Here's how the part is built. I have some questions about the finished solid (model axes, mm). Face numbers are marked on the shaded views. A direction names the side the tool comes from. Give positions to 0.01 mm unless a question says otherwise; leave off trailing zeros. Order: outer loops, then holes, each group sorted by start corner. A loop starts at its lowest first (then second) coordinate and runs counter-clockwise, first axis right, second up. Notation, with made-up numbers: (70, 52) - (96, 52) arc R27 cw to (96, 90) - close; hole circle Ø11 at (72.25, 69). An arc over 180 degrees is marked (long way). One line per question, with ' | ' between items.
from build123d import *

# Parameters (mm, degrees)
SKETCH1_R               = 6.477
BOSS_EXTRUDE2_DEPTH     = 12.7
CUT_EXTRUDE1_DEPTH      = 2.032
CUT_EXTRUDE1_TAPER      = 15
CUT_EXTRUDE2_DEPTH      = 2.032
CUT_EXTRUDE2_TAPER      = 15
SKETCH6_R               = 15.308441
SKETCH6_R_2             = 10.16
CUT_EXTRUDE3_DEPTH      = 112.76
CUT_EXTRUDE3_DEPTH_BACK = 11.16


with BuildPart() as part:
    # Sketch1 → Boss-Extrude2 (new body)
    with BuildSketch(Plane.XY):
        with BuildLine():
            Line((-10.16, 0), (-10.16, 12.7))
            Line((-10.16, 12.7), (-3.181447, 28.448))
            Line((-3.181447, 28.448), (-3.181447, 91.950959))
            ThreePointArc((-3.181447, 91.950959), (0, 111.76), (3.181447, 91.950959))
            Line((3.181447, 91.950959), (3.181447, 28.448))
            Line((3.181447, 28.448), (10.16, 12.7))
            Line((10.16, 12.7), (10.16, 0))
            ThreePointArc((10.16, 0), (0, -10.16), (-10.16, 0))
        make_face()
        Circle(SKETCH1_R, mode=Mode.SUBTRACT)
        with Locations((0, 101.6)):
            Circle(SKETCH1_R, mode=Mode.SUBTRACT)
    extrude(amount=BOSS_EXTRUDE2_DEPTH)

    # Sketch3 → Cut-Extrude1 (cut)
    with BuildSketch(Plane.XY.offset(12.7)):
        with BuildLine():
            ThreePointArc((-0.895447, 89.408), (-1.973078, 88.961631), (-2.419447, 87.884))
            Line((-2.419447, 87.884), (-2.419447, 32.766))
            ThreePointArc((-2.419447, 32.766), (-1.973078, 31.688369), (-0.895447, 31.242))
            Line((-0.895447, 31.242), (0.895447, 31.242))
            ThreePointArc((0.895447, 31.242), (1.973078, 31.688369), (2.419447, 32.766))
            Line((2.419447, 32.766), (2.419447, 87.884))
            ThreePointArc((2.419447, 87.884), (1.973078, 88.961631), (0.895447, 89.408))
            Line((0.895447, 89.408), (-0.895447, 89.408))
        make_face()
    extrude(amount=-CUT_EXTRUDE1_DEPTH, taper=CUT_EXTRUDE1_TAPER, mode=Mode.SUBTRACT)

    # Sketch5 → Cut-Extrude2 (cut)
    with BuildSketch(Plane(origin=(0, 0, 0), x_dir=(-1, 0, 0), z_dir=(0, 0, -1))):
        with BuildLine():
            ThreePointArc((-0.895447, 89.408), (-1.973078, 88.961631), (-2.419447, 87.884))
            Line((-2.419447, 87.884), (-2.419447, 32.766))
            ThreePointArc((-2.419447, 32.766), (-1.973078, 31.688369), (-0.895447, 31.242))
            Line((-0.895447, 31.242), (0.895447, 31.242))
            ThreePointArc((0.895447, 31.242), (1.973078, 31.688369), (2.419447, 32.766))
            Line((2.419447, 32.766), (2.419447, 87.884))
            ThreePointArc((2.419447, 87.884), (1.973078, 88.961631), (0.895447, 89.408))
            Line((0.895447, 89.408), (-0.895447, 89.408))
        make_face()
    extrude(amount=-CUT_EXTRUDE2_DEPTH, taper=CUT_EXTRUDE2_TAPER, mode=Mode.SUBTRACT)

    # Sketch6 → Cut-Extrude3 (cut, two sides)
    with BuildSketch(Plane(origin=(0, 0, 0), x_dir=(1, 0, 0), z_dir=(0, 1, 0))) as cut_extrude3_sk:
        with Locations((0, -6.388373)):
            Circle(SKETCH6_R)
        with Locations((0, -6.388373)):
            Circle(SKETCH6_R_2, mode=Mode.SUBTRACT)
    extrude(amount=CUT_EXTRUDE3_DEPTH, mode=Mode.SUBTRACT)
    extrude(cut_extrude3_sk.sketch, amount=-CUT_EXTRUDE3_DEPTH_BACK, mode=Mode.SUBTRACT)


solid = part.part
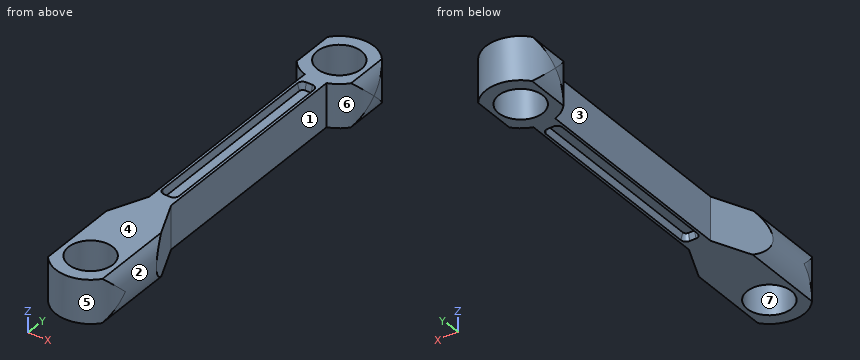
1) Please list where these lines run through material, in increasing order: L1, parallel to Y at x = 0, z = 7.75; L2, parallel to Y at x = 4.5, z = 1; L3, parallel to Y at x = 4, z = 5.
Model answer:
L1: y = -10.16 to -6.48, 6.48 to 95.12, 108.08 to 111.76 | L2: y = -9.11 to -4.66, 4.66 to 25.47, 92.49 to 96.94, 106.26 to 110.71 | L3: y = -9.34 to -5.09, 5.09 to 26.6, 92.26 to 96.51, 106.69 to 110.94
2) I'm going to push flat-ended pins straight in: P1, Ø4, axis at y = 51.5, z = 7.5, coming from the -X side; P2, Ø1.9, axis at x = -0.5, y = 49.5, coming from the -Z side; P3, Ø4, axis at x = 8, z = 10.5, coming from the +Y side. Where does each tip first touch, or does it pass through?
Model answer:
P1: stops at x = -3.18 | P2: stops at z = 2.03 | P3: stops at y = 109.8
3) I want a section at B-B (z = 5). List the corners of the cut face in (x, y) for me, plus the area to 3 significant figures.
Model answer:
outline: (-10.06, -1.39) arc R10.16 ccw to (10.06, -1.39) - (10.06, 12.92) - (3.18, 28.45) - (3.18, 91.95) arc R10.16 ccw to (10.06, 100.21) - (10.06, 102.99) arc R10.16 ccw to (-10.06, 102.99) - (-10.06, 100.21) arc R10.16 ccw to (-3.18, 91.95) - (-3.18, 28.45) - (-10.06, 12.92) - close; hole circle Ø12.95 at (0, 0); hole circle Ø12.95 at (0, 101.6) | area: 1,090 mm2
4) I want a section at C-C (y = 21). List the corners of the cut face in (x, z) for me.
Model answer:
outline: (-6.48, 0) - (6.48, 0) - (6.48, 12.7) - (-6.48, 12.7) - close
5) I want a section at A-A (y = 96.5). List the corners of the cut face in (x, z) for me.
Model answer:
outline: (-8.79, 1.29) arc R10.16 ccw to (-7.9, 0) - (-3.99, 0) - (-3.99, 12.7) - (-7.96, 12.7) arc R10.16 ccw to (-8.79, 11.49) - close; (3.99, 0) - (7.9, 0) arc R10.16 ccw to (8.79, 1.29) - (8.79, 11.49) arc R10.16 ccw to (7.96, 12.7) - (3.99, 12.7) - close
6) On a 3-axis mill with a long thin cutter (end or side, diameter ignored), from which of +Z, -Z, +X, -X, +Y, -Y can I reach the whole of each face in a straight line? I mean the marked faces 1, 2 and 3. Say none if no direction works.
Model answer:
face 1: +Z, -Z, +X | face 2: +X, +Y, -Y | face 3: +Z, -Z, -X
7) Thinking about a two-plate mould opening in X: for the marked faces 4, 5, 6 and 7, which applies, +X half, -X half, draft (parallel to the pull), parting line (faces both ways), or undercut?
Model answer:
face 4: draft | face 5: parting line | face 6: +X half | face 7: undercut
